Job drawing, mm, ordinate dimensions from the low corner. One solid piece. A direction names the side the tool comes from. Round coordinates to 2 decimals unless told otherwise and drop trailing zeros. Loops run counter-clockwise (first coordinate to the right, second up) from the corner with the lowest first, then second, coordinate; pieces in that order, holes last. Notation, with made-up numbers: M 1,89.5 L 12,89.5 A29 cw 12,125.5 Z; hole C 49.5,78.25 d1. An arc over 180 degrees is marked long. Use a Markdown table: item, result. Add a question column.
(1) Wall check: L1, parallel to Y at x = 13, z = 45.5; L2, parallel to Z at x = 45, y = 14; L3, parallel to X at y = 11.5, z = 5.5. Give the ranges that are in metal, low to high.
(2) Which spindle directions (+Z, -Z, +X, -X, +Y, -Y) get a long thin tool onto all of the face, cutting with end or side? Do the marked faces 1, 2, 3 and 4. Say none if no direction does.
(3) Two-plate mould, pull along Y, no slides. Class the marked faces 5, 6 and 7: released by +Y, released by -Y, zero draft, split by the parting line, or undercut.
(4) Band-saw the part on C-C, the plane y = 13.5. Write the cut outline in (x, z).
(5) Flat gauge pins, fed straight in: P1, Ø5, axis at y = 10, z = 6.5, coming from the +X side; P2, Ø9, axis at y = 15, z = 15, coming from the +X side; P3, Ø2, axis at x = 44, y = 22, coming from the -Z side. Where does each tip first touch, or does it go through?
(6) Band-saw the part on D-D, the plane x = 10. Write the cut outline in (y, z), and give its area (3 significant figures).
(7) Band-saw the part on B-B, the plane z = 13. Write the cut outline in (x, y), and give its area (3 significant figures).
(8) Band-saw the part on A-A, the plane x = 83. Write the cut outline in (y, z), and give its area (3 significant figures).
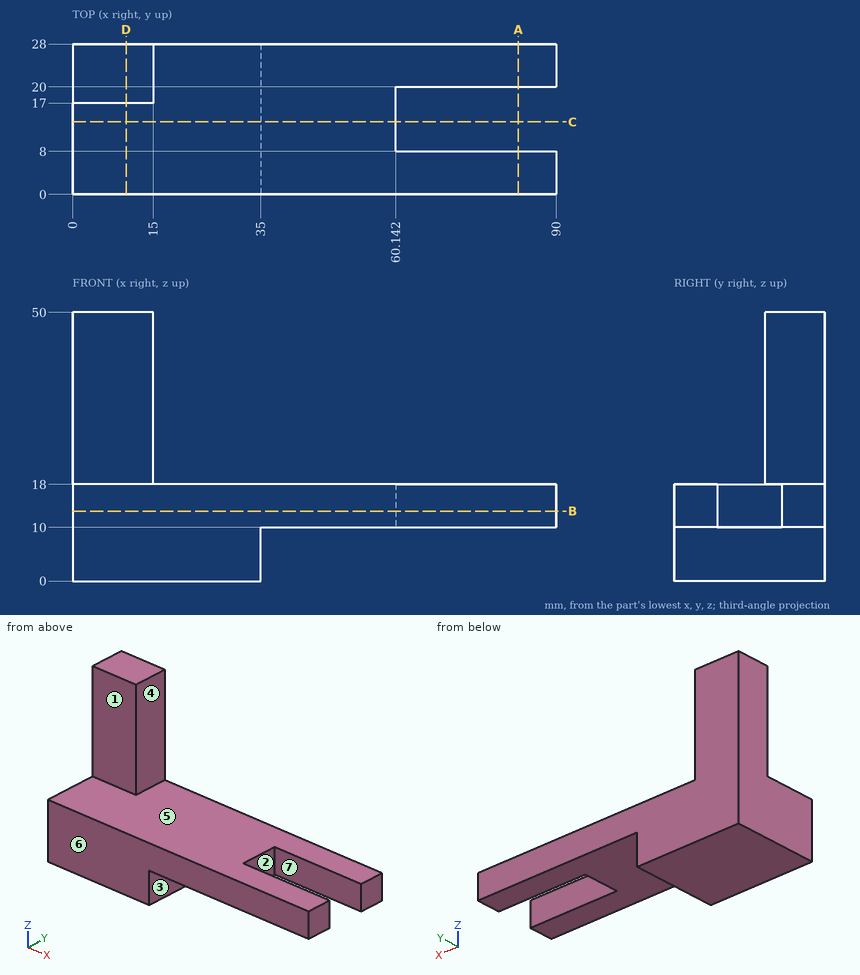
Return value:
| question | item | result |
|---|---|---|
| 1 | L1 | 17 to 28 |
| 1 | L2 | 10 to 18 |
| 1 | L3 | 0 to 35 |
| 2 | face 1 | +Z, +X, -X, -Y |
| 2 | face 2 | +Z, -Z, +X |
| 2 | face 3 | -Z, +X, +Y, -Y |
| 2 | face 4 | +Z, +X, +Y, -Y |
| 3 | face 5 | zero draft |
| 3 | face 6 | released by -Y |
| 3 | face 7 | undercut |
| 4 | outline | M 0,0 L 35,0 L 35,10 L 60.14,10 L 60.14,18 L 0,18 Z |
| 5 | P1 | x = 35 |
| 5 | P2 | x = 60.14 |
| 5 | P3 | z = 10 |
| 6 | outline | M 0,0 L 28,0 L 28,50 L 17,50 L 17,18 L 0,18 Z |
| 6 | area | 856 mm^2 |
| 7 | outline | M 0,0 L 90,0 L 90,8 L 60.14,8 L 60.14,20 L 90,20 L 90,28 L 0,28 Z |
| 7 | area | 2,160 mm^2 |
| 8 | outline | M 0,10 L 8,10 L 8,18 L 0,18 Z; M 20,10 L 28,10 L 28,18 L 20,18 Z |
| 8 | area | 128 mm^2 |
